Build history of the part. All positions in model axes, mm. Face numbers are marked on the shaded views. A direction names the side the tool comes from. Round coordinates to 2 decimals unless told otherwise and drop trailing zeros. Write each loop counter-clockwise with the first axis right and the second up, starting at its lowest first coordinate (ties: lowest second). Pieces come first, ordered by that corner, then holes. Notation, with made-up numbers: (-27.75, 11.5) -> (8.25, 11.5) arc R30 ccw to (8.25, 34.5) -> close; hole circle Ø11 at (-18, 62). An arc over 180 degrees is marked (long way). Answer in a Markdown table with one row per item.
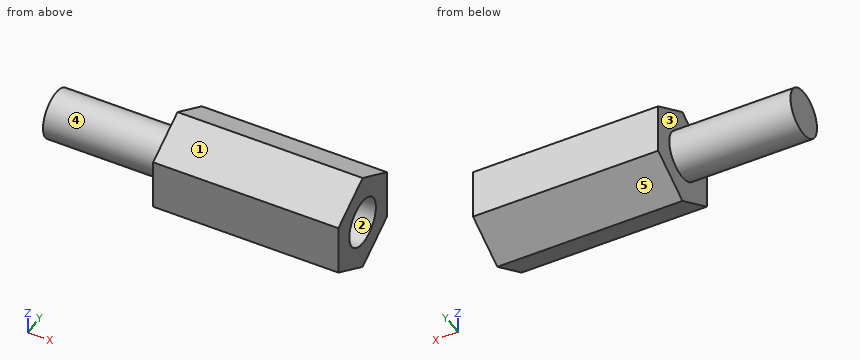
Autodesk Inventor part; units mm, degrees
ref_plane "YZ Plane" through (0, 0, 0) normal (1, 0, 0) x (0, 1, 0)
ref_plane "XZ Plane" through (0, 0, 0) normal (0, 1, 0) x (-1, 0, 0)
ref_plane "XY Plane" through (0, 0, 0) normal (0, 0, 1) x (1, 0, 0)
sketch "Sketch1" plane through (0, 0, 0) normal (1, 0, 0) x (0, 1, 0)
  line L0 (0.0055, 3.1659) -> (2.7555, 1.5782)
  line L1 (2.7555, 1.5782) -> (2.7555, -1.5973)
  line L2 (2.7555, -1.5973) -> (0.0055, -3.185)
  line L3 (0.0055, -3.185) -> (-2.7445, -1.5973)
  line L4 (-2.7445, -1.5973) -> (-2.7445, 1.5782)
  line L5 (-2.7445, 1.5782) -> (0.0055, 3.1659)
  point P0 (0.0055, -0.0095)
  dimension "d1" = 5.5
extrude "Extrusion1" add sketch "Sketch1" along normal blind 11.639
sketch "Sketch2" plane through (0, 0, 0) normal (-1, 0, 0) x (0, 0, 1)
  circle A0 centre (0, 0) radius 1.5
  dimension "d4" = 3
extrude "Extrusion2" add sketch "Sketch2" along normal blind 7.619
sketch "Sketch3" plane through (11.639, 0, 0) normal (1, 0, 0) x (0, 0, -1)
  circle A0 centre (0, 0) radius 1.5
  dimension "d7" = 3
extrude "Extrusion3" cut sketch "Sketch3" against normal blind 6
properties part number "Spacer" material "Brass, Soft Yellow"
Q1. Which spindle directions (+Z, -Z, +X, -X, +Y, -Y) get a long thin tool onto all of the face, cutting with end or side? Do the marked faces 4 and 5. Say none if no direction does.
A:
| item | result |
|---|---|
| face 4 | -X |
| face 5 | -Z, +X, -X, +Y |
Q2. Saw through at A-A on x = 9.5. Write the cut outline in (y, z) (1 decimal).
A:
| item | result |
|---|---|
| outline | (-2.7, -1.6) -> (0, -3.2) -> (2.8, -1.6) -> (2.8, 1.6) -> (0, 3.2) -> (-2.7, 1.6) -> close; hole circle Ø3 at (0, 0) |
Q3. Two-plate mould, pull along Z, no slides. Class the marked faces 1, 2 and 3: released by +Z, released by -Z, zero draft, split by the parting line, or undercut.
A:
| item | result |
|---|---|
| face 1 | released by +Z |
| face 2 | undercut |
| face 3 | zero draft |
Q4. Drop flat-ended pins along their axis: P1, Ø0.9, axis at y = 0, z = -0.5, coming from the +X side; P2, Ø1.5, axis at x = 3.5, y = -2, coming from the -Z side; P3, Ø1.5, axis at x = -5, z = 1.5, coming from the +Y side. Give the stop position or say it passes through.
A:
| item | result |
|---|---|
| P1 | x = 5.64 |
| P2 | z = -2.46 |
| P3 | y = 1.3 |
Q5. Saw through at C-C on y = 0.85. Write the cut outline in (x, z), plus the area to 3 significant figures.
A:
| item | result |
|---|---|
| outline | (-7.62, -1.24) -> (0, -1.24) -> (0, -2.7) -> (11.64, -2.7) -> (11.64, -1.24) -> (5.64, -1.24) -> (5.64, 1.24) -> (11.64, 1.24) -> (11.64, 2.68) -> (0, 2.68) -> (0, 1.24) -> (-7.62, 1.24) -> close |
| area | 66.6 mm² |
Q6. Wall check: line 1 (Y direction, x = 7.8, z = 0); line 2 (X direction, y = -0.65, z = 1.25); line 3 (X direction, y = 0.25, z = -2). Give the ranges that are in metal, low to high. Write a range as [from, to].
A:
| item | result |
|---|---|
| line 1 | [-2.74, -1.5], [1.5, 2.76] |
| line 2 | [-7.62, 5.64] |
| line 3 | [0, 11.64] |
Q7. Saw through at D-D on z = 1.75. Write the cut outline in (x, y).
A:
| item | result |
|---|---|
| outline | (0, -2.45) -> (11.64, -2.45) -> (11.64, 2.46) -> (0, 2.46) -> close |
Q8. Saw through at B-B on z = 0. Write the cut outline in (x, y), plus the area to 3 significant figures.
A:
| item | result |
|---|---|
| outline | (-7.62, -1.5) -> (0, -1.5) -> (0, -2.74) -> (11.64, -2.74) -> (11.64, -1.5) -> (5.64, -1.5) -> (5.64, 1.5) -> (11.64, 1.5) -> (11.64, 2.76) -> (0, 2.76) -> (0, 1.5) -> (-7.62, 1.5) -> close |
| area | 68.9 mm² |
